```python
from build123d import *

# Parameters (mm, degrees)
BOSS_EXTRUDE1_DEPTH = 10.16
FILLET1_R           = 2.54
SKETCH3_R           = 1.651
CUT_EXTRUDE1_DEPTH  = 10.16
FILLET2_R           = 0.254


with BuildPart() as part:
    # Sketch2 → Boss-Extrude1 (new body)
    with BuildSketch(Plane.XY):
        Polygon((12.7, 13.894017094), (-12.7, 13.894017094), (-12.7, 5.334), (-25.019, 5.334), (-25.019, 0), (-5.969, 0), (-5.969, 9.877777778), (5.969, 9.877777778), (5.969, 0), (25.019, 0), (25.019, 5.334), (12.7, 5.334), align=None)
    extrude(amount=BOSS_EXTRUDE1_DEPTH)

    # Fillet1
    fillet1_edges = [part.edges().sort_by_distance(p)[0] for p in [
        (-12.7, 13.894017094, 5.08),
        (12.7, 13.894017094, 5.08),
        (-25.019, 2.667, 10.16),
        (25.019, 2.667, 10.16),
    ]]
    fillet(fillet1_edges, radius=FILLET1_R)

    # Sketch3 → Cut-Extrude1 (cut)
    with BuildSketch(Plane(origin=(0, 0, 0), x_dir=(1, 0, 0), z_dir=(0, 1, 0))):
        with Locations((-19.558, -5.296219795)):
            Circle(SKETCH3_R)
        with Locations((19.558, -5.296219795)):
            Circle(SKETCH3_R)
    extrude(amount=CUT_EXTRUDE1_DEPTH, mode=Mode.SUBTRACT)

    # Fillet2
    fillet2_edges = [part.edges().sort_by_distance(p)[0] for p in [
        (5.969, 9.877777778, 5.08),
        (-5.969, 9.877777778, 5.08),
    ]]
    fillet(fillet2_edges, radius=FILLET2_R)


solid = part.part
```
Model file for the job. Use its own axes, mm. A direction names the side the tool comes from. Round coordinates to 2 decimals unless told otherwise and drop trailing zeros. Order: outer loops, then holes, each group sorted by start corner. A loop starts at its lowest first (then second) coordinate and runs counter-clockwise, first axis right, second up. Notation, with made-up numbers: M -35.5,4.25 L 16.5,4.25 A23 cw 16.5,35.25 Z; hole C -4,22.25 d2. An arc over 180 degrees is marked long. Use CSV: the item, a comma, the result in double quotes.
Item 1: Saw through at D-D (x = 19.5). List the corners of the cut face in (y, z).
Worked answers:
outline,"M 0,0 L 5.33,0 L 5.33,3.65 L 0,3.65 Z; M 0,6.95 L 5.33,6.95 L 5.33,10.16 L 0,10.16 Z"
Item 2: Pin check, flat tips, straight feed: pin 1 (1 mm diameter, centred on y = 8.5, z = 4, fed in from +X); pin 2 (3 mm diameter, centred on y = 8.5, z = 6.5, fed in from -X); pin 3 (5 mm diameter, centred on x = -18.5, z = 7.5, fed in from +Y); pin 4 (2 mm diameter, centred on x = -19.56, z = 5.3, fed in from -Y). Stop position of each tip, or through.
Worked answers:
pin 1,"x = 12.7"
pin 2,"x = -12.7"
pin 3,"y = 5.33"
pin 4,"through"
Item 3: Which spindle directions (+Z, -Z, +X, -X, +Y, -Y) get a long thin tool onto all of the face, cutting with end or side? Do faces 1 (the face through (-24.29, 2.63, 9.4)), 2 (the face through (-12.7, 8, 5)), 3 (the face through (0, 13.894, 5)), 4 (the face through (17.6, 5.334, 5)), 5 (the face through (-5.969, 5, 5)). Say none if no direction does.
Worked answers:
face 1,"+Z, -X, +Y, -Y"
face 2,"+Z, -Z, -X, +Y"
face 3,"+Z, -Z, +X, -X, +Y"
face 4,"+Z, -Z, +X, +Y"
face 5,"+Z, -Z, -Y"
Item 4: Saw through at A-A (y = 7.75). List the corners of the cut face in (x, z).
Worked answers:
outline,"M -12.7,0 L -5.97,0 L -5.97,10.16 L -12.7,10.16 Z; M 5.97,0 L 12.7,0 L 12.7,10.16 L 5.97,10.16 Z"
Item 5: Probe probe 1 along X at (y, z) = (2.5, 1); probe 2 along X at (y, z) = (7.25, 8.75); probe 3 along X at (y, z) = (10, 8.75). List the from-to ranges inside material, lowest first.
Worked answers:
probe 1,"-25.02 to -5.97, 5.97 to 25.02"
probe 2,"-12.7 to -5.97, 5.97 to 12.7"
probe 3,"-12.7 to 12.7"
Item 6: Saw through at C-C (y = 2). List the corners of the cut face in (x, z).
Worked answers:
outline,"M -25.02,0 L -5.97,0 L -5.97,10.16 L -22.48,10.16 A2.54 ccw -25.02,7.62 Z; M 5.97,0 L 25.02,0 L 25.02,7.62 A2.54 ccw 22.48,10.16 L 5.97,10.16 Z; hole C -19.56,5.3 d3.3; hole C 19.56,5.3 d3.3"
Item 7: Pull direction Z, two halves, no side cores. Call faces 6 (the face through (-18.033, 2.63, 5.929)), 7 (the face through (-0.3, 10.1, 10.16)), 8 (the face through (-11.936, 13.17, 5.151)): released by +Z, released by -Z, zero draft, split by the parting line, or undercut.
Worked answers:
face 6,"undercut"
face 7,"released by +Z"
face 8,"zero draft"
Item 8: Saw through at B-B (z = 6.5). List the corners of the cut face in (x, y) (3 decimals).
Worked answers:
outline,"M -25.019,0 L -20.688,0 L -20.688,5.334 L -25.019,5.334 Z; M -18.428,0 L -5.969,0 L -5.969,9.624 A0.254 cw -5.715,9.878 L 5.715,9.878 A0.254 cw 5.969,9.624 L 5.969,0 L 18.428,0 L 18.428,5.334 L 12.7,5.334 L 12.7,11.354 A2.54 ccw 10.16,13.894 L -10.16,13.894 A2.54 ccw -12.7,11.354 L -12.7,5.334 L -18.428,5.334 Z; M 20.688,0 L 25.019,0 L 25.019,5.334 L 20.688,5.334 Z"
